Input: part model. Units: mm. Frame: model coordinates. Give positions to 0.01 mm unless a question says otherwise; leave off trailing zeros. Loops run counter-clockwise (first coordinate to the right, second up) from the corner with the lowest first, then second, coordinate; pieces in that order, holes last. Notation, with made-up numbers: (73.5, 20) - (116.5, 20) arc R32 ccw to (116.5, 49) - close; hole circle Ø7 at (57, -1). An arc over 180 degrees is marked (long way). Answer as a JSON object with one key per item and string values. Group by question number.
(1) Material intervals for L1, parallel to Z at x = -1.5, y = -2.25; L2, parallel to Z at x = -1.25, y = 0.5; L3, parallel to X at y = 1.5, z = -4.25, sorted ascending.
(2) Section query A-A (x = 0). Return loops of the section in (y, z) (3 decimals), plus the area to 3 significant figures.
(3) Pin query (flat end, axial travel): P1, Ø1.5, axis at x = 1, z = 7.5, coming from the +Y side. Return the tip coordinate at first contact, or that it passes through.
(4) Section query B-B (z = -1.5). Return loops of the section in (x, y) (3 decimals).
```python
from build123d import *

# Parameters (mm, degrees)
SKETCH1_R           = 3.835
BOSS_EXTRUDE1_DEPTH = 14
SKETCH2_R           = 2.25
BOSS_EXTRUDE2_DEPTH = 2
FILLET1_R           = 1


with BuildPart() as part:
    # Sketch1 → Boss-Extrude1 (new, symmetric)
    with BuildSketch(Plane.XY):
        Circle(SKETCH1_R)
    extrude(amount=BOSS_EXTRUDE1_DEPTH, both=True)

    # Sketch2 → Boss-Extrude2 (add)
    with BuildSketch(Plane(origin=(0, 0, -14), x_dir=(-1, 0, 0), z_dir=(0, 0, -1))):
        Circle(SKETCH2_R)
    extrude(amount=BOSS_EXTRUDE2_DEPTH)

    # Fillet1
    fillet1_edges = [part.edges().sort_by_distance(p)[0] for p in [
        (-3.835, 0, -14),
        (-3.835, 0, 14),
        (2.25, 0, -16),
    ]]
    fillet(fillet1_edges, radius=FILLET1_R)


solid = part.part
```
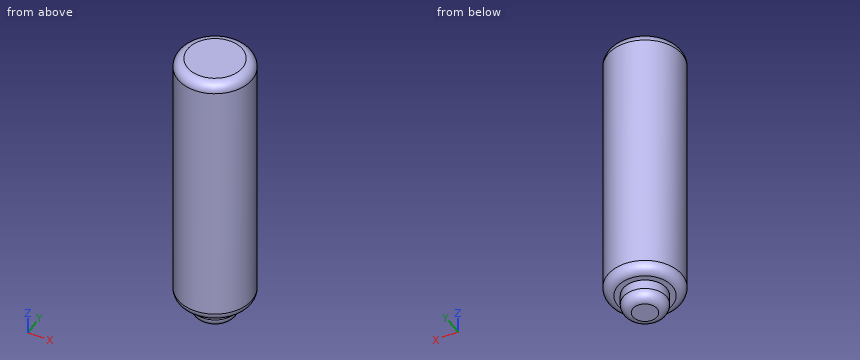
Recorded:
{
 "1": {"L1": "z = -14 to 14", "L2": "z = -16 to 14", "L3": "x = -3.53 to 3.53"},
 "2": {"outline": "(-3.835, -13) arc R1 ccw to (-2.835, -14) - (-2.25, -14) - (-2.25, -15) arc R1 ccw to (-1.25, -16) - (1.25, -16) arc R1 ccw to (2.25, -15) - (2.25, -14) - (2.835, -14) arc R1 ccw to (3.835, -13) - (3.835, 13) arc R1 ccw to (2.835, 14) - (-2.835, 14) arc R1 ccw to (-3.835, 13) - close", "area": "222 mm^2"},
 "3": {"P1": "stops at y = 3.83"},
 "4": {"outline": "circle Ø7.67 at (0, 0)"}
}
